Solid Edge part; units mm, degrees
sketch "Sketch1" plane through (0, 0, 0) normal (0, 0, 1) x (1, 0, 0)
  circle A0 centre (0, 0) radius 2.725
extrude "Protrusion1" add sketch "Sketch1" against normal blind 3
sketch "Sketch2" plane through (0, 0, 0) normal (0, 0, 1) x (1, 0, 0)
  line L0 (-0.7, -1.2124) -> (-1.05, -0.6062)
  line L1 (-1.4, 0) -> (-1.05, -0.6062)
  line L2 (-1.4, 0) -> (-1.05, 0.6062)
  line L3 (-0.7, 1.2124) -> (-1.05, 0.6062)
  line L4 (-0.7, 1.2124) -> (0, 1.2124)
  line L5 (0.7, 1.2124) -> (0, 1.2124)
  line L6 (0.7, 1.2124) -> (1.05, 0.6062)
  line L7 (1.4, 0) -> (1.05, 0.6062)
  line L8 (1.4, 0) -> (1.05, -0.6062)
  line L9 (0.7, -1.2124) -> (1.05, -0.6062)
  line L10 (0.7, -1.2124) -> (0, -1.2124)
  line L11 (-0.7, -1.2124) -> (0, -1.2124)
extrude "ExtrudedCutout_1" cut sketch "Sketch2" against normal blind 1.45
sketch "Sketch3" plane through (0, 0, -3) normal (0, 0, -1) x (1, 0, 0)
  circle A0 centre (0, 0) radius 1.5
extrude "ExtrudedProtrusion_2" add sketch "Sketch3" along normal blind 30
cosmetic_thread "Thread_2" thread depth 17
Build history of the part. All positions in model axes, mm. A direction names the side the tool comes from. Round coordinates to 2 decimals unless told otherwise and drop trailing zeros. Write each loop counter-clockwise with the first axis right and the second up, starting at its lowest first coordinate (ties: lowest second). Pieces come first, ordered by that corner, then holes. Notation, with made-up numbers: M -3.75,-11 L 14.25,-11 A15 cw 14.25,-4 Z; hole C 86.5,41 d3. An arc over 180 degrees is marked long. Use CSV: the item, a comma, the result in double quotes.
1. Saw through at A-A (x = 0). Give the cut face in (y, z) (3 decimals), plus the area to 3 significant figures.
Reply:
outline,"M -2.725,-3 L -1.5,-3 L -1.5,-33 L 1.5,-33 L 1.5,-3 L 2.725,-3 L 2.725,0 L 1.212,0 L 1.212,-1.45 L -1.212,-1.45 L -1.212,0 L -2.725,0 Z"
area,"103 mm²"
2. Two-plate mould, pull along X, no slides. Class faces 1 (the face through (1, -1, 0)), 2 (the face through (0, -1.212, -1)), 3 (the face through (-1.5, 0.07, -17.79)), 4 (the face through (-1.05, 0.61, -0.71)): +X half, -X half, draft (parallel to the pull), parting line (faces both ways), or undercut.
Reply:
face 1,"draft"
face 2,"undercut"
face 3,"parting line"
face 4,"undercut"
3. Tool access for faces 5 (the face through (2.6, 0.82, -1.48)), 6 (the face through (1.2, -1.2, -3)), 7 (the face through (1.055, 0.598, -0.715)): list every direction of +Z, -Z, +X, -X, +Y, -Y with a clear straight run to the whole face (end or side of a thin tool).
Reply:
face 5,"+Z, -Z"
face 6,"-Z"
face 7,"+Z"
4. Flat gauge pins, fed straight in: pin 1 (0.7 mm diameter, centred on x = 0, y = 0, fed in from +Z); pin 2 (3 mm diameter, centred on y = 1, z = -24, fed in from -X); pin 3 (1.5 mm diameter, centred on y = 1.5, z = -29, fed in from +X). Where does each tip first touch, or does it go through?
Reply:
pin 1,"stops at z = -1.45"
pin 2,"stops at x = -1.5"
pin 3,"stops at x = 1.3"
5. Saw through at B-B (z = -3.5). Give the cut face in (x, y), plus the area to 3 significant figures.
Reply:
outline,"C 0,0 d3"
area,"7.07 mm²"
6. Saw through at D-D (x = -2.15). Give the cut face in (y, z), plus the area to 3 significant figures.
Reply:
outline,"M -1.67,-3 L 1.67,-3 L 1.67,0 L -1.67,0 Z"
area,"10.0 mm²"
7. Wall check: probe 1 along Z at (x, y) = (-1.55, -1.25); probe 2 along Z at (x, y) = (-0.7, -0.2); probe 3 along Y at (x, z) = (0, -11). Give the ranges that are in metal, low to high. Write a range as from..to.
Reply:
probe 1,"z = -3..0"
probe 2,"z = -33..-1.45"
probe 3,"y = -1.5..1.5"
8. Saw through at C-C (x = 2). Give the cut face in (y, z), plus the area to 3 significant figures.
Reply:
outline,"M -1.85,-3 L 1.85,-3 L 1.85,0 L -1.85,0 Z"
area,"11.1 mm²"
